Build history of the part. All positions in model axes, mm. A direction names the side the tool comes from. Give positions to 0.01 mm unless a question says otherwise; leave off trailing zeros. Order: outer loops, then holes, each group sorted by start corner. A loop starts at its lowest first (then second) coordinate and runs counter-clockwise, first axis right, second up. Notation, with made-up numbers: (16, 32.5) -> (62, 32.5) arc R20 ccw to (62, 59.5) -> close; hole circle Ø4 at (-13.75, 82). An arc over 180 degrees is marked (long way). One line per item, written item: value. Start each with the question number.
(1) Probe line 1 (Z direction, x = 198, y = 0); line 2 (Z direction, x = 94.5, y = -4). List the from-to ranges inside material, lowest first.
(2) Two-plate mould, pull along Z, no slides. Class faces 5 (the conical face through (310.28, 9.28, -12.11)), 6 (the cylindrical face through (52.5, 11.59, -15.12)), 7 (the flat face through (330, -16, 6)): +Z half, -Z half, draft (parallel to the pull), parting line (faces both ways), or undercut.
(3) Saw through at A-A on z = 0. Give the cut face in (x, y), plus the area to 3 significant figures.
(4) Pin check, flat tips, straight feed: pin 1 (6 mm diameter, centred on x = 141, y = -0.5, fed in from -Z); pin 2 (2 mm diameter, centred on x = 116.5, y = 4, fed in from +Z); pin 3 (15 mm diameter, centred on y = 0, z = 0, fed in from -X); pin 4 (6 mm diameter, centred on x = 195.5, z = 7.5, fed in from +Y). Stop position of each tip, or through.
(5) Saw through at C-C on x = 104.5. Give the cut face in (y, z).
(6) Saw through at D-D on x = 306.5. Give the cut face in (y, z).
(7) Which spindle directions (+Z, -Z, +X, -X, +Y, -Y) get a long thin tool onto all of the face, cutting with end or side? Do faces 1 (the cylindrical face through (306.86, 11.59, -15.12)), 2 (the flat face through (30, -16, -6)), 3 (the flat face through (290, 11.32, -6.14)), 4 (the cylindrical face through (178.6, -4.959, 15.748)). Say none if no direction does.
```python
from build123d import *


# Not quite as in the source:
# - a fillet or chamfer that OpenCascade refuses, or shapes differently, is made with other operations: its cross-section is extruded or revolved along the edge and cut away or added


with BuildPart() as f2:
    # F0 (on Front) → F2 (revolve)
    with BuildSketch(Plane.XZ):
        Polygon((0, 15.24), (0, 12.7), (30, 12.7), (290, 12.7), (290, 13.97), (330, 16.51), (330, 19.05), (280, 19.05), (280, 16.51), (80, 16.51), (80, 19.05), (30, 19.05), (30, 16.51), align=None)
    revolve(axis=Axis((0, 0, 0), (1, 0, 0)))

    # F3: fillet of radius 5 on 2 edges, made by hand

    # F3_s1 → F3_t2 (revolve, cut)
    with BuildSketch(Plane.XZ):
        with BuildLine():
            ThreePointArc((80, 16.51), (78.1669446402, 18.3685645763), (75.6470240065, 19.05))
            Line((75.6470240065, 19.05), (75.6470240065, 19.15))
            Line((75.6470240065, 19.15), (80, 19.15))
            Line((80, 19.15), (80.1, 19.05))
            ThreePointArc((80.1, 19.05), (80.1, 17.78), (80.0870595199, 16.5592))
            Line((80.0870595199, 16.5592), (80, 16.51))
        make_face()
    revolve(axis=Axis((80, 0, 0), (1, 0, 0)), mode=Mode.SUBTRACT)

    # F3_s3 → F3_t4 (revolve, cut)
    with BuildSketch(Plane.XZ):
        with BuildLine():
            ThreePointArc((284.3529759935, 19.05), (281.8330553598, 18.3685645763), (280, 16.51))
            Line((280, 16.51), (279.9129404801, 16.5592))
            ThreePointArc((279.9129404801, 16.5592), (279.9, 17.78), (279.9, 19.05))
            Line((279.9, 19.05), (280, 19.15))
            Line((280, 19.15), (284.3529759935, 19.15))
            Line((284.3529759935, 19.15), (284.3529759935, 19.05))
        make_face()
    revolve(axis=Axis((280, 0, 0), (1, 0, 0)), mode=Mode.SUBTRACT)


solid = f2.part
```
Results below:
1. line 1: z = -16.51 to -12.7, 12.7 to 16.51
1. line 2: z = -16.02 to -12.05, 12.05 to 16.02
2. face 5: undercut
2. face 6: parting line
2. face 7: draft
3. outline: (0, -15.24) -> (30, -16.51) -> (30, -19.05) -> (75.65, -19.05) arc R5 ccw to (80, -16.51) -> (280, -16.51) arc R5 ccw to (284.35, -19.05) -> (330, -19.05) -> (330, -16.51) -> (290, -13.97) -> (290, -12.7) -> (0, -12.7) -> close; (0, 12.7) -> (290, 12.7) -> (290, 13.97) -> (330, 16.51) -> (330, 19.05) -> (284.35, 19.05) arc R5 ccw to (280, 16.51) -> (80, 16.51) arc R5 ccw to (75.65, 19.05) -> (30, 19.05) -> (30, 16.51) -> (0, 15.24) -> close
3. area: 2,770 mm²
4. pin 1: stops at z = -16.51
4. pin 2: stops at z = 16.24
4. pin 3: passes through
4. pin 4: stops at y = 15.88
5. outline: circle Ø33.02 at (0, 0); hole circle Ø25.4 at (0, 0)
6. outline: circle Ø38.1 at (0, 0); hole circle Ø30.04 at (0, 0)
7. face 1: +X, -X
7. face 2: -X
7. face 3: +X
7. face 4: none
